from build123d import *

# Parameters (mm, degrees)
F3_DEPTH = 48


with BuildPart() as f1:
    # F0 (on Right) → F1 (revolve)
    with BuildSketch(Plane.YZ):
        Polygon((37.5, 0), (0, 0), (0, -7), (31, -7), (31, -35.75), (34, -35.75), (34, -75.75), (35.5, -75.75), (35.5, -80.75), (37.5, -80.75), (37.5, -21.75), (33.5, -21.75), (33.5, -18.75), (37.5, -18.75), (37.5, -14.75), (33.9, -14.75), (33.9, -12.75), (37.5, -12.75), (37.5, -8.75), (34.5, -8.75), (34.5, -7), (37.5, -7), align=None)
    revolve(axis=Axis((0, 0, -21.27509), (0, 0, -1)))

    # F2 (on face) → F3 (join)
    with BuildSketch(Plane(origin=(0, 0, -80.75), x_dir=(1, 0, 0), z_dir=(0, 0, -1))):
        with BuildLine():
            Line((-30, -22.5), (-30, 22.5))
            ThreePointArc((-30, 22.5), (-37.5, 0), (-30, -22.5))
        make_face()
        with BuildLine():
            ThreePointArc((30, -22.5), (37.5, 0), (30, 22.5))
            Line((30, 22.5), (30, -22.5))
        make_face()
    extrude(amount=-F3_DEPTH)


solid = f1.part
Verification items for the finished model (mm, model axes). A direction names the side the tool comes from. Coordinates: 2 decimals unless noted, no trailing zeros. Order: outer loops, then holes, each group sorted by start corner. A loop starts at its lowest first (then second) coordinate and runs counter-clockwise, first axis right, second up. Notation, with made-up numbers: (-30.5, 71.5) -> (9.5, 71.5) arc R35 ccw to (9.5, 104.5) -> close; hole circle Ø11 at (-10, -27.75). An arc over 180 degrees is marked (long way). Put each result on its own line as item: value. Start each with the question number.
1. Material ranges on L1, parallel to Z at x = 27, y = -25; L2, parallel to Z at x = 24.5, y = -23; L3, parallel to X at y = 0, z = -13, recorded low to high. Write a range as [from, to].
2. Go/stop test with flat-tipped pins: pin 1 Ø10 at (x, y) = (-25, 20.5) entering from +Z; pin 2 Ø5 at (y, z) = (-7, -53.5) entering from -X; pin 3 Ø12 at (x, z) = (-16, -41) entering from -Y; pin 4 Ø11.5 at (y, z) = (-0.5, -57) entering from -X. Record where each tip stops, or that it passes through.
3. Mould release check, pull along X, two halves, no side actions. Record for faces 1 (the flat face through (1, -1, 0)), 2 (the cylindrical face through (37.18, -4.88, -3.45)), 3 (the cylindrical face through (-0.5, 35.496, -78.285)): released by +X, released by -X, zero draft, split by the parting line, or undercut.
4. Cross-section at A-A, the plane z = -45.5. Record the boundary of the cut face in (x, y).
5. Access from +Z, -Z, +X, -X, +Y, -Y to the whole of each face (thin tool, end or side, straight path). Record for faces 4 (the flat face through (30, 0, -57)), 5 (the cylindrical face through (10.363, 32.907, -7.863)), 6 (the cylindrical face through (37.18, -4.88, -10.72)).
6. Cross-section at B-B, the plane z = -24. Record the boundary of the cut face in (x, y).
Computed:
1. L1: [-80.75, -21.75], [-18.75, -14.75], [-12.75, -8.75], [-7, 0]
1. L2: [-35.75, -21.75], [-18.75, 0]
1. L3: [-33.9, -31], [31, 33.9]
2. pin 1: z = 0
2. pin 2: x = -37.23
2. pin 3: y = -36.14
2. pin 4: x = -37.5
3. face 1: zero draft
3. face 2: split by the parting line
3. face 3: undercut
4. outline: circle Ø75 at (0, 0); hole (-30, -16) arc R34 ccw to (30, -16) -> (30, 16) arc R34 ccw to (-30, 16) -> close
5. face 4: -Z
5. face 5: none
5. face 6: +Z, -Z
6. outline: circle Ø75 at (0, 0); hole circle Ø62 at (0, 0)
